from build123d import *

# Parameters (mm, degrees)
SKETCH_1_R               = 1.5
EXTRUDE_1_DEPTH          = 10
CUT_EXTRUDE_1_DEPTH      = 52.14684741
CUT_EXTRUDE_1_DEPTH_BACK = 52.14684741
SKETCH_3_R               = 3
SKETCH_3_W               = 5
SKETCH_3_H               = 10
CHAMFER_1_SIZE           = 3.5


with BuildPart() as part:
    # 草图1 → 凸台-拉伸1 (new, symmetric)
    with BuildSketch(Plane(origin=(0, 0, 0), x_dir=(0, 0, -1), z_dir=(1, 0, 0))):
        with BuildLine():
            Line((0, -4), (-44.803847577, -4))
            Line((-44.803847577, -4), (-50, -1))
            Line((-50, -1), (-50, 0))
            Line((-50, 0), (-4, 0))
            ThreePointArc((-4, 0), (2.828427125, 2.828427125), (0, -4))
        make_face()
        Circle(SKETCH_1_R, mode=Mode.SUBTRACT)
    extrude(amount=EXTRUDE_1_DEPTH, both=True)

    # 草图3 → 切除-拉伸1 (cut, two sides: drawn at the far end of the back side and taken through both)
    with BuildSketch(Plane(origin=(0, 0, 0), x_dir=(1, 0, 0), z_dir=(0, 1, 0)).offset(-CUT_EXTRUDE_1_DEPTH_BACK)):
        with Locations(Location((0, -35, 0), (0, 0, 270))):
            Circle(SKETCH_3_R)
        with Locations((-7.5, -1)):
            Rectangle(SKETCH_3_W, SKETCH_3_H)
        with Locations((7.5, -1)):
            Rectangle(SKETCH_3_W, SKETCH_3_H)
    extrude(amount=CUT_EXTRUDE_1_DEPTH + CUT_EXTRUDE_1_DEPTH_BACK, mode=Mode.SUBTRACT)

    # 倒角1
    chamfer_1_edges = [part.edges().sort_by_distance(p)[0] for p in [
        (0, 0, 32),
    ]]
    chamfer(chamfer_1_edges, length=CHAMFER_1_SIZE)


solid = part.part
Read the model definition and answer for the solid it produces. Units are mm, in the model's axes. A direction names the side the tool comes from. Coordinates: 2 decimals unless noted, no trailing zeros. Loops run counter-clockwise (first coordinate to the right, second up) from the corner with the lowest first, then second, coordinate; pieces in that order, holes last.
Q1. Consider probe 1 along Z at (x, y) = (3.75, -1.25); probe 2 along X at (y, z) = (-3.8, 35); probe 3 along Y at (x, z) = (7, 44.5). Determine where each line is inside the solid, lowest interval first.
Q2. The part is cut by section B-B on z = 35. Write down the section's boundary in (x, y), and give its area (4 significant figures).
Q3. Which of the six approach directions +Z, -Z, +X, -X, +Y, -Y give full straight-line access (tool end or side, diameter ignored) to faces 4 (the face through (-5, -1, 2)), 5 (the face through (0.1, -2.5, 47.4)), 6 (the face through (7, -2, 6))?
Q4. Each of these flat-tipped pins is pushed along its axis until it touches: pin 1 Ø4.5 at (x, y) = (7, -2.5) entering from -Z; pin 2 Ø1.5 at (x, z) = (2.5, 15) entering from +Y; pin 3 Ø2 at (y, z) = (2, 42.5) entering from +X; pin 4 Ø1 at (x, z) = (0, 3.5) entering from +Y. Where does it stop, or does it pass through?
Q5. The part is cut by section C-C on y = -0.5. Write down the section's boundary in (x, z), and give its area (3 significant figures).
Q6. The part is cut by section D-D on x = 7.75. Write down the section's boundary in (y, z).
Q7. The mould has two halves that part along Z. Classify faces 1 (the face through (0, 0, 27)), 2 (the face through (0.1, -0.5, 50)), 3 (the face through (1.233, -3.281, 37.973)): +Z half, -Z half, draft (parallel to the pull), parting line (faces both ways), or undercut.
Q8. The part is cut by section A-A on x = 0. Write down the section's boundary in (y, z).
Results below:
1. probe 1: z = -3.8 to -0.83, 0.83 to 31.33, 38.67 to 49.57
1. probe 2: x = -10 to -3, 3 to 10
1. probe 3: y = -4 to 0
2. outline: (-10, -4) - (-3, -4) - (-3, -3.5) - (-6.5, 0) - (-10, 0) - close; (3, -4) - (10, -4) - (10, 0) - (6.5, 0) - (3, -3.5) - close
2. area: 43.75 mm2
3. face 4: -Z, -X, +Y, -Y
3. face 5: +Z, +X, -X, -Y
3. face 6: -Z, +X, +Y, -Y
4. pin 1: stops at z = -3.72
4. pin 2: stops at y = 0
4. pin 3: passes through
4. pin 4: stops at y = 2.65
5. outline: (-10, 6) - (-5, 6) - (-5, 1.41) - (5, 1.41) - (5, 6) - (10, 6) - (10, 50) - (-10, 50) - close; (-5, -3.97) - (5, -3.97) - (5, -1.41) - (-5, -1.41) - close; hole circle Ø12 at (0, 35)
5. area: 838 mm2
6. outline: (-4, 6) - (0, 6) - (0, 50) - (-1, 50) - (-4, 44.8) - close
7. face 1: draft
7. face 2: +Z half
7. face 3: undercut
8. outline: (-4, 0) arc R4 ccw (long way) to (0, 4) - (0, 28.5) - (-3.5, 32) - (-4, 32) - close; (-4, 38) - (-3.5, 38) - (0, 41.5) - (0, 50) - (-1, 50) - (-4, 44.8) - close; hole circle Ø3 at (0, 0)
